Job drawing, mm, ordinate dimensions from the low corner. One solid piece. A direction names the side the tool comes from. Round coordinates to 2 decimals unless told otherwise and drop trailing zeros. Order: outer loops, then holes, each group sorted by start corner. A loop starts at its lowest first (then second) coordinate and runs counter-clockwise, first axis right, second up. Notation, with made-up numbers: (67, 16.5) -> (75, 16.5) arc R15 cw to (75, 30.5) -> close; hole circle Ø8 at (-13, 72). An arc over 180 degrees is marked (long way). Return JSON: item names as keys, results as strings. Group by question number.
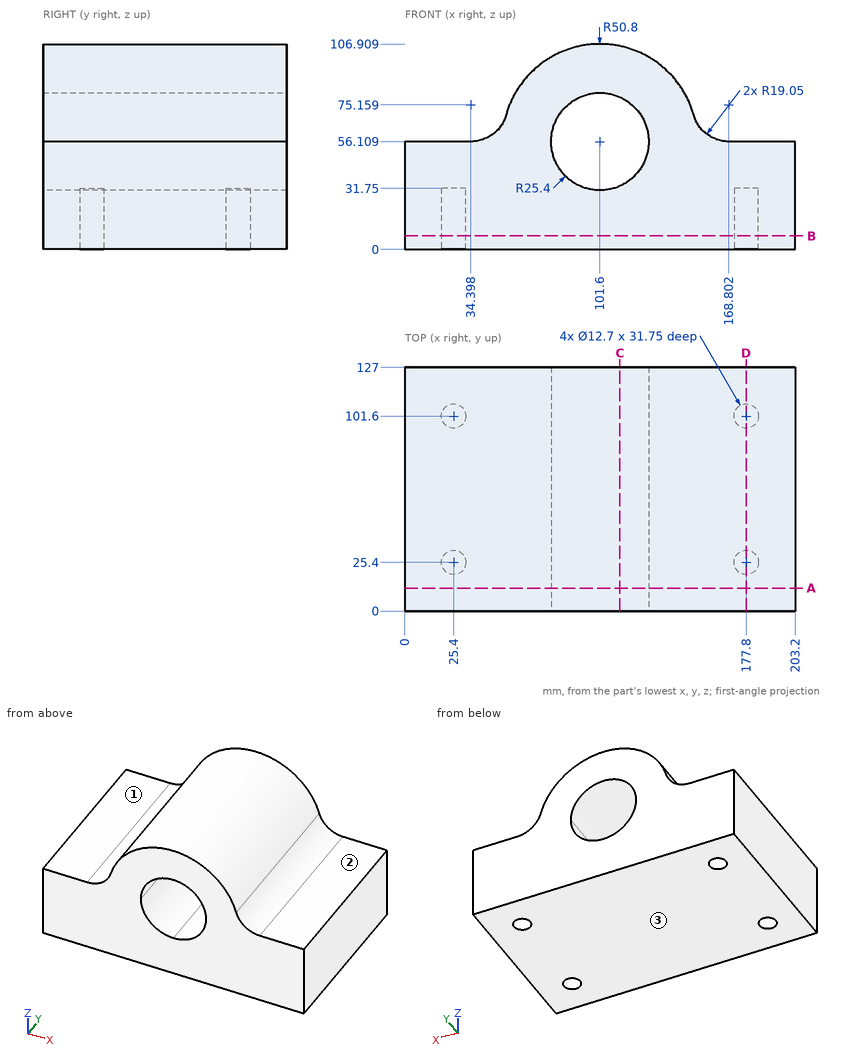
(1) Pin check, flat tips, straight feed: P1, Ø7.5, axis at x = 25.4, y = 101.6, coming from the -Z side; P2, Ø2, axis at x = 144.5, y = 14, coming from the -Z side; P3, Ø7.5, axis at x = 177.8, y = 25.4, coming from the +Z side; P4, Ø4, axis at x = 126.5, y = 109, coming from the +Z side. Stop position of each tip, or through.
(2) Saw through at C-C, the plane x = 112. List the corners of the cut face in (y, z).
(3) Probe L1, parallel to X at y = 25, z = 18; L2, parallel to Y at x = 177, z = 15; L3, parallel to Z at x = 86, y = 53. List the from-to ranges inside material, lowest first. Write a range as [from, to].
(4) Saw through at A-A, the plane y = 12. List the corners of the cut face in (x, z).
(5) Saw through at D-D, the plane x = 177.8. List the corners of the cut face in (y, z).
(6) Tool access for the marked faces 1, 2 and 3: list every direction of +Z, -Z, +X, -X, +Y, -Y with a clear straight run to the whole face (end or side of a thin tool).
(7) Saw through at B-B, the plane z = 7. List the corners of the cut face in (x, y).
Results are:
{
 "1": {"P1": "stops at z = 31.75", "P2": "stops at z = 0", "P3": "stops at z = 56.11", "P4": "stops at z = 101.45"},
 "2": {"outline": "(0, 0) -> (127, 0) -> (127, 32.94) -> (0, 32.94) -> close; (0, 79.28) -> (127, 79.28) -> (127, 105.83) -> (0, 105.83) -> close"},
 "3": {"L1": "x = [0, 19.06], [31.74, 171.46], [184.14, 203.2]", "L2": "y = [0, 19.1], [31.7, 95.3], [107.9, 127]", "L3": "z = [0, 36.06], [76.15, 104.45]"},
 "4": {"outline": "(0, 0) -> (203.2, 0) -> (203.2, 56.11) -> (168.8, 56.11) arc R19.05 cw to (150.47, 69.96) arc R50.8 ccw to (52.73, 69.96) arc R19.05 cw to (34.4, 56.11) -> (0, 56.11) -> close; hole circle Ø50.8 at (101.6, 56.11)"},
 "5": {"outline": "(0, 0) -> (19.05, 0) -> (19.05, 31.75) -> (31.75, 31.75) -> (31.75, 0) -> (95.25, 0) -> (95.25, 31.75) -> (107.95, 31.75) -> (107.95, 0) -> (127, 0) -> (127, 56.11) -> (0, 56.11) -> close"},
 "6": {"face 1": "+Z, -X, +Y, -Y", "face 2": "+Z, +X, +Y, -Y", "face 3": "-Z, +X, -X, +Y, -Y"},
 "7": {"outline": "(0, 0) -> (203.2, 0) -> (203.2, 127) -> (0, 127) -> close; hole circle Ø12.7 at (25.4, 25.4); hole circle Ø12.7 at (25.4, 101.6); hole circle Ø12.7 at (177.8, 25.4); hole circle Ø12.7 at (177.8, 101.6)"}
}
